Verification items for the finished model (mm, model axes). Face numbers are marked on the shaded views. Round coordinates to 2 decimals unless told otherwise and drop trailing zeros. Order: outer loops, then holes, each group sorted by start corner. A loop starts at its lowest first (then second) coordinate and runs counter-clockwise, first axis right, second up. Notation, with made-up numbers: M 33.5,-5 L 64.5,-5 A9 ccw 64.5,4 Z; hole C 41,-33 d3. An arc over 180 degrees is marked long. Use CSV: the item, a comma, the result in double quotes. Start each with the question number.
Q1. Sectioned sample at B-B (x = 39). Enter the section's corners in (y, z), and give its area (3 significant figures).
Q2. Sectioned sample at D-D (y = -22.5). Enter the section's corners in (x, z).
Q3. Scan lines: line 1 (Y direction, x = -45, z = 89); line 2 (X direction, y = -8.5, z = 50). Record each from-to range of solid material in increasing order.
Q4. Gauge pin test, flat ends, axial feed: pin 1 Ø2 at (y, z) = (-60.5, 89) entering from -X; pin 2 Ø5 at (x, y) = (-27, -2) entering from +Z; pin 3 Ø5 at (y, z) = (-131.5, 31.5) entering from -X. Record the tip position at first contact, or that the pin passes through.
Q5. Mould release check, pull along Y, two halves, no side actions. Record for the marked faces 1, 2, 3 and 4: +Y half, -Y half, draft (parallel to the pull), parting line (faces both ways), or undercut.
Q6. Sectioned sample at A-A (z = 49). Enter the section's corners in (x, y), and give its area (3 significant figures).
Q7. Sectioned sample at C-C (z = 80). Enter the section's corners in (x, y), and give its area (3 significant figures).
```python
from build123d import *

# Parameters (mm, degrees)
F0_R     = 1.651
F1_DEPTH = 133.9596
F3_DEPTH = 123.825
F4_R     = 50.8
F5_R     = 1.5
F6_DEPTH = 25.4


with BuildPart() as f1:
    # F0 (on Front) → F1 (new body)
    with BuildSketch(Plane.XZ):
        Polygon((-34.6942804754, 11.2792461441), (-34.6942804754, 53.1892461441), (-24.0262804754, 53.1892461441), (-24.0262804754, 103.3542461441), (-74.8262804754, 103.3542461441), (-74.8262804754, -14.1207538559), (-24.0262804754, -14.1207538559), (-24.0262804754, 11.2792461441), align=None)
        with Locations((-29.2570274323, 7.2342461441)):
            Circle(F0_R, mode=Mode.SUBTRACT)
        with Locations((-29.2570274323, 57.2342461441)):
            Circle(F0_R, mode=Mode.SUBTRACT)
        Polygon((-24.0262804754, 103.3542461441), (-24.0262804754, 53.1892461441), (-13.3582804754, 53.1892461441), (-13.3582804754, 11.2792461441), (-24.0262804754, 11.2792461441), (-24.0262804754, -14.1207538559), (55.3487195246, -14.1207538559), (55.3487195246, 103.3542461441), align=None)
        with Locations((-19.2570274323, 7.2342461441)):
            Circle(F0_R, mode=Mode.SUBTRACT)
        with Locations((-19.2570274323, 57.2342461441)):
            Circle(F0_R, mode=Mode.SUBTRACT)
    extrude(amount=F1_DEPTH)

    # F2 (on face) → F3 (cut)
    with BuildSketch(Plane(origin=(-74.8262804754, 0, 0), x_dir=(0, -1, 0), z_dir=(-1, 0, 0))):
        Polygon((127.6096, 103.3542461441), (6.35, 103.3542461441), (6.35, -14.1207538559), (111.6725547834, -14.1207538559), (127.6096, -14.1207538559), align=None)
    extrude(amount=-F3_DEPTH, mode=Mode.SUBTRACT)

    # F4
    f4_edges = [f1.edges().sort_by_distance(p)[0] for p in [
        (-74.82628, -130.7846, -14.120754),
        (-74.82628, -130.7846, 103.354246),
        (-74.82628, -3.175, -14.120754),
        (-74.82628, -3.175, 103.354246),
    ]]
    fillet(f4_edges, radius=F4_R)

    # F5 (on face) → F6 (cut)
    with BuildSketch(Plane.YZ.offset(55.3487195246)):
        with BuildLine():
            ThreePointArc((-116.2798, 44.6167461441), (-116.7191398282, 45.6774063159), (-117.7798, 46.1167461441))
            Line((-117.7798, 46.1167461441), (-117.7798, 43.1167461441))
            ThreePointArc((-117.7798, 43.1167461441), (-116.7191398282, 43.5560859723), (-116.2798, 44.6167461441))
        make_face()
        with BuildLine():
            Line((-117.7798, 43.1167461441), (-117.7798, 46.1167461441))
            ThreePointArc((-117.7798, 46.1167461441), (-119.2798, 44.6167461441), (-117.7798, 43.1167461441))
        make_face()
        with Locations((-92.3798, 44.6167461441)):
            Circle(F5_R)
        with Locations((-66.9798, 44.6167461441)):
            Circle(F5_R)
        with Locations((-41.5798, 44.6167461441)):
            Circle(F5_R)
        with BuildLine():
            Line((-16.1798, 43.1167461441), (-16.1798, 46.1167461441))
            ThreePointArc((-16.1798, 46.1167461441), (-17.6798, 44.6167461441), (-16.1798, 43.1167461441))
        make_face()
        with BuildLine():
            ThreePointArc((-14.6798, 44.6167461441), (-15.1191398282, 45.6774063159), (-16.1798, 46.1167461441))
            Line((-16.1798, 46.1167461441), (-16.1798, 43.1167461441))
            ThreePointArc((-16.1798, 43.1167461441), (-15.1191398282, 43.5560859723), (-14.6798, 44.6167461441))
        make_face()
        with BuildLine():
            Line((-16.1798, 17.7167461441), (-16.1798, 20.7167461441))
            ThreePointArc((-16.1798, 20.7167461441), (-17.6798, 19.2167461441), (-16.1798, 17.7167461441))
        make_face()
        with BuildLine():
            ThreePointArc((-14.6798, 19.2167461441), (-15.1191398282, 20.2774063159), (-16.1798, 20.7167461441))
            Line((-16.1798, 20.7167461441), (-16.1798, 17.7167461441))
            ThreePointArc((-16.1798, 17.7167461441), (-15.1191398282, 18.1560859723), (-14.6798, 19.2167461441))
        make_face()
        with Locations((-41.5798, 19.2167461441)):
            Circle(F5_R)
        with Locations((-66.9798, 19.2167461441)):
            Circle(F5_R)
        with Locations((-92.3798, 19.2167461441)):
            Circle(F5_R)
        with BuildLine():
            Line((-117.7798, 17.7167461441), (-117.7798, 20.7167461441))
            ThreePointArc((-117.7798, 20.7167461441), (-119.2798, 19.2167461441), (-117.7798, 17.7167461441))
        make_face()
        with BuildLine():
            Line((-117.7798, -6.1832538559), (-117.7798, -4.6832538559))
            ThreePointArc((-117.7798, -4.6832538559), (-118.8404601718, -7.2439140277), (-116.2798, -6.1832538559))
            Line((-116.2798, -6.1832538559), (-117.7798, -6.1832538559))
        make_face()
        with BuildLine():
            ThreePointArc((-116.2798, 19.2167461441), (-116.7191398282, 20.2774063159), (-117.7798, 20.7167461441))
            Line((-117.7798, 20.7167461441), (-117.7798, 17.7167461441))
            ThreePointArc((-117.7798, 17.7167461441), (-116.7191398282, 18.1560859723), (-116.2798, 19.2167461441))
        make_face()
        with BuildLine():
            ThreePointArc((-90.8798, -6.1832538559), (-92.3798, -4.6832538559), (-93.8798, -6.1832538559))
            Line((-93.8798, -6.1832538559), (-90.8798, -6.1832538559))
        make_face()
        with BuildLine():
            Line((-90.8798, -6.1832538559), (-93.8798, -6.1832538559))
            ThreePointArc((-93.8798, -6.1832538559), (-92.3798, -7.6832538559), (-90.8798, -6.1832538559))
        make_face()
        with BuildLine():
            ThreePointArc((-65.4798, -6.1832538559), (-66.9798, -4.6832538559), (-68.4798, -6.1832538559))
            Line((-68.4798, -6.1832538559), (-65.4798, -6.1832538559))
        make_face()
        with BuildLine():
            Line((-65.4798, -6.1832538559), (-68.4798, -6.1832538559))
            ThreePointArc((-68.4798, -6.1832538559), (-66.9798, -7.6832538559), (-65.4798, -6.1832538559))
        make_face()
        with BuildLine():
            ThreePointArc((-40.0798, -6.1832538559), (-41.5798, -4.6832538559), (-43.0798, -6.1832538559))
            Line((-43.0798, -6.1832538559), (-40.0798, -6.1832538559))
        make_face()
        with BuildLine():
            Line((-40.0798, -6.1832538559), (-43.0798, -6.1832538559))
            ThreePointArc((-43.0798, -6.1832538559), (-41.5798, -7.6832538559), (-40.0798, -6.1832538559))
        make_face()
        with BuildLine():
            ThreePointArc((-14.6798, -6.1832538559), (-15.1191398282, -5.1225936841), (-16.1798, -4.6832538559))
            Line((-16.1798, -4.6832538559), (-16.1798, -6.1832538559))
            Line((-16.1798, -6.1832538559), (-17.6798, -6.1832538559))
            ThreePointArc((-17.6798, -6.1832538559), (-16.1798, -7.6832538559), (-14.6798, -6.1832538559))
        make_face()
        with BuildLine():
            Line((-16.1798, -6.1832538559), (-16.1798, -4.6832538559))
            ThreePointArc((-16.1798, -4.6832538559), (-17.2404601718, -5.1225936841), (-17.6798, -6.1832538559))
            Line((-17.6798, -6.1832538559), (-16.1798, -6.1832538559))
        make_face()
        with BuildLine():
            ThreePointArc((-116.2798, -6.1832538559), (-116.7191398282, -5.1225936841), (-117.7798, -4.6832538559))
            Line((-117.7798, -4.6832538559), (-117.7798, -6.1832538559))
            Line((-117.7798, -6.1832538559), (-116.2798, -6.1832538559))
        make_face()
        with BuildLine():
            ThreePointArc((-116.2798, 70.0167461441), (-116.7191398282, 71.0774063159), (-117.7798, 71.5167461441))
            Line((-117.7798, 71.5167461441), (-117.7798, 68.5167461441))
            ThreePointArc((-117.7798, 68.5167461441), (-116.7191398282, 68.9560859723), (-116.2798, 70.0167461441))
        make_face()
        with BuildLine():
            Line((-117.7798, 68.5167461441), (-117.7798, 71.5167461441))
            ThreePointArc((-117.7798, 71.5167461441), (-119.2798, 70.0167461441), (-117.7798, 68.5167461441))
        make_face()
        with Locations((-92.3798, 70.0167461441)):
            Circle(F5_R)
        with Locations((-66.9798, 70.0167461441)):
            Circle(F5_R)
        with Locations((-41.5798, 70.0167461441)):
            Circle(F5_R)
        with BuildLine():
            ThreePointArc((-14.6798, 70.0167461441), (-15.1191398282, 71.0774063159), (-16.1798, 71.5167461441))
            Line((-16.1798, 71.5167461441), (-16.1798, 68.5167461441))
            ThreePointArc((-16.1798, 68.5167461441), (-15.1191398282, 68.9560859723), (-14.6798, 70.0167461441))
        make_face()
        with BuildLine():
            Line((-16.1798, 68.5167461441), (-16.1798, 71.5167461441))
            ThreePointArc((-16.1798, 71.5167461441), (-17.6798, 70.0167461441), (-16.1798, 68.5167461441))
        make_face()
        with BuildLine():
            ThreePointArc((-14.6798, 95.4167461441), (-16.1798, 96.9167461441), (-17.6798, 95.4167461441))
            Line((-17.6798, 95.4167461441), (-16.1798, 95.4167461441))
            Line((-16.1798, 95.4167461441), (-16.1798, 93.9167461441))
            ThreePointArc((-16.1798, 93.9167461441), (-15.1191398282, 94.3560859723), (-14.6798, 95.4167461441))
        make_face()
        with BuildLine():
            Line((-16.1798, 95.4167461441), (-17.6798, 95.4167461441))
            ThreePointArc((-17.6798, 95.4167461441), (-17.2404601718, 94.3560859723), (-16.1798, 93.9167461441))
            Line((-16.1798, 93.9167461441), (-16.1798, 95.4167461441))
        make_face()
        with BuildLine():
            ThreePointArc((-40.0798, 95.4167461441), (-41.5798, 96.9167461441), (-43.0798, 95.4167461441))
            Line((-43.0798, 95.4167461441), (-40.0798, 95.4167461441))
        make_face()
        with BuildLine():
            Line((-40.0798, 95.4167461441), (-43.0798, 95.4167461441))
            ThreePointArc((-43.0798, 95.4167461441), (-41.5798, 93.9167461441), (-40.0798, 95.4167461441))
        make_face()
        with BuildLine():
            Line((-65.4798, 95.4167461441), (-68.4798, 95.4167461441))
            ThreePointArc((-68.4798, 95.4167461441), (-66.9798, 93.9167461441), (-65.4798, 95.4167461441))
        make_face()
        with BuildLine():
            ThreePointArc((-65.4798, 95.4167461441), (-66.9798, 96.9167461441), (-68.4798, 95.4167461441))
            Line((-68.4798, 95.4167461441), (-65.4798, 95.4167461441))
        make_face()
        with BuildLine():
            ThreePointArc((-90.8798, 95.4167461441), (-92.3798, 96.9167461441), (-93.8798, 95.4167461441))
            Line((-93.8798, 95.4167461441), (-90.8798, 95.4167461441))
        make_face()
        with BuildLine():
            Line((-117.7798, 95.4167461441), (-116.2798, 95.4167461441))
            ThreePointArc((-116.2798, 95.4167461441), (-118.8404601718, 96.4774063159), (-117.7798, 93.9167461441))
            Line((-117.7798, 93.9167461441), (-117.7798, 95.4167461441))
        make_face()
        with BuildLine():
            ThreePointArc((-117.7798, 93.9167461441), (-116.7191398282, 94.3560859723), (-116.2798, 95.4167461441))
            Line((-116.2798, 95.4167461441), (-117.7798, 95.4167461441))
            Line((-117.7798, 95.4167461441), (-117.7798, 93.9167461441))
        make_face()
        with BuildLine():
            Line((-90.8798, 95.4167461441), (-93.8798, 95.4167461441))
            ThreePointArc((-93.8798, 95.4167461441), (-92.3798, 93.9167461441), (-90.8798, 95.4167461441))
        make_face()
    extrude(amount=-F6_DEPTH, mode=Mode.SUBTRACT)


solid = f1.part
```
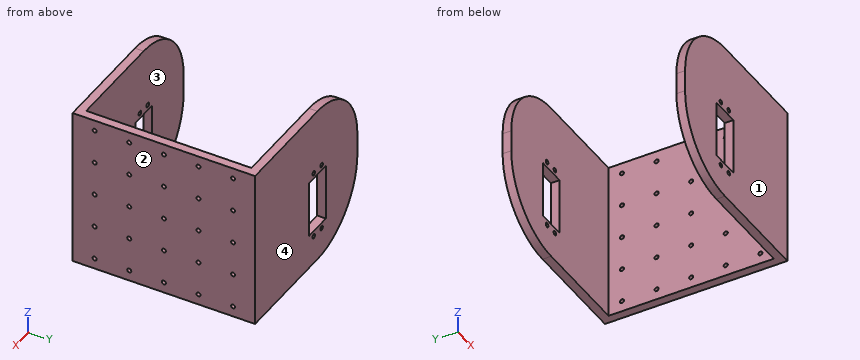
Verdict:
1,outline,"M -133.96,-14.12 L -127.61,-14.12 L -127.61,103.35 L -133.96,103.35 Z; M -6.35,-14.12 L 0,-14.12 L 0,103.35 L -6.35,103.35 Z"
1,area,"1,490 mm²"
2,outline,"M 49,-14.12 L 55.35,-14.12 L 55.35,103.35 L 49,103.35 Z"
3,line 1,"y = -133.96 to -127.61, -6.35 to 0"
3,line 2,"x = 49 to 55.35"
4,pin 1,"stops at x = 49"
4,pin 2,"stops at z = 103.35"
4,pin 3,"stops at x = -74.76"
5,face 1,"-Y half"
5,face 2,"draft"
5,face 3,"undercut"
5,face 4,"+Y half"
6,outline,"M -74.83,-133.96 L -34.69,-133.96 L -34.69,-127.61 L -74.83,-127.61 Z; M -74.83,-6.35 L -34.69,-6.35 L -34.69,0 L -74.83,0 Z; M -13.36,-133.96 L 55.35,-133.96 L 55.35,0 L -13.36,0 L -13.36,-6.35 L 49,-6.35 L 49,-127.61 L -13.36,-127.61 Z"
6,area,"2,150 mm²"
7,outline,"M -66.77,-133.96 L 55.35,-133.96 L 55.35,0 L -66.77,0 L -66.77,-6.35 L 49,-6.35 L 49,-127.61 L -66.77,-127.61 Z"
7,area,"2,320 mm²"
